The model under review builds one solid part; all positions refer to its coordinate system, in mm. Round coordinates to 2 decimals unless told otherwise and drop trailing zeros.
```python
from build123d import *

# Parameters (mm, degrees)
SKETCH3_R           = 2.201333333
SKETCH3_R_2         = 1.693333333
BOSS_EXTRUDE1_DEPTH = 914.4
CUT_EXTRUDE1_DEPTH  = 733.425


with BuildPart() as part:
    # Sketch3 → Boss-Extrude1 (new, symmetric)
    with BuildSketch(Plane.XY):
        with BuildLine():
            Line((-1.778, 0), (-1.778, 1.27))
            ThreePointArc((-1.778, 1.27), (-1.536070654, 2.494011801), (-0.846666667, 3.533942971))
            Line((-0.846666667, 3.533942971), (2.413267273, 6.793876912))
            ThreePointArc((2.413267273, 6.793876912), (2.578074335, 6.903997469), (2.772477518, 6.942666667))
            Line((2.772477518, 6.942666667), (3.048, 6.942666667))
            ThreePointArc((3.048, 6.942666667), (3.467078619, 6.769078619), (3.640666667, 6.35))
            Line((3.640666667, 6.35), (3.640666667, 4.301066667))
            ThreePointArc((3.640666667, 4.301066667), (3.948165494, 3.558698827), (4.690533333, 3.2512))
            Line((4.690533333, 3.2512), (5.300133333, 3.2512))
            ThreePointArc((5.300133333, 3.2512), (6.042501173, 3.558698827), (6.35, 4.301066667))
            Line((6.35, 4.301066667), (6.35, 10.583333333))
            ThreePointArc((6.35, 10.583333333), (5.730042687, 12.080042687), (4.233333333, 12.7))
            Line((4.233333333, 12.7), (-4.233333333, 12.7))
            ThreePointArc((-4.233333333, 12.7), (-5.730042687, 12.080042687), (-6.35, 10.583333333))
            Line((-6.35, 10.583333333), (-6.35, 0))
            Line((-6.35, 0), (-1.778, 0))
        make_face()
        with Locations(Location((-2.116666667, 8.466666667, 0), (0, 0, 180))):
            Circle(SKETCH3_R, mode=Mode.SUBTRACT)
        with Locations(Location((3.429, 9.906, 0), (0, 0, 180))):
            Circle(SKETCH3_R_2, mode=Mode.SUBTRACT)
    extrude(amount=BOSS_EXTRUDE1_DEPTH, both=True)

    # Mirror1: part across plane


with BuildPart() as part_1:
    add(part.part)
    add(part.part.mirror(Plane.ZX))

    # Sketch4 → Cut-Extrude1 (cut)
    with BuildSketch(Plane.XY.offset(914.4)):
        with BuildLine():
            Line((-6.35, 10.583333333), (-6.35, -10.583333333))
            ThreePointArc((-6.35, -10.583333333), (-5.730042687, -12.080042687), (-4.233333333, -12.7))
            Line((-4.233333333, -12.7), (4.233333333, -12.7))
            ThreePointArc((4.233333333, -12.7), (5.730042687, -12.080042687), (6.35, -10.583333333))
            Line((6.35, -10.583333333), (6.35, -4.301066667))
            ThreePointArc((6.35, -4.301066667), (6.042501173, -3.558698827), (5.300133333, -3.2512))
            Line((5.300133333, -3.2512), (4.690533333, -3.2512))
            ThreePointArc((4.690533333, -3.2512), (3.948165494, -3.558698827), (3.640666667, -4.301066667))
            Line((3.640666667, -4.301066667), (3.640666667, -6.35))
            ThreePointArc((3.640666667, -6.35), (3.467078619, -6.769078619), (3.048, -6.942666667))
            Line((3.048, -6.942666667), (2.772477518, -6.942666667))
            ThreePointArc((2.772477518, -6.942666667), (2.578074335, -6.903997469), (2.413267273, -6.793876912))
            Line((2.413267273, -6.793876912), (-0.846666667, -3.533942971))
            ThreePointArc((-0.846666667, -3.533942971), (-1.536070654, -2.494011801), (-1.778, -1.27))
            Line((-1.778, -1.27), (-1.778, 1.27))
            ThreePointArc((-1.778, 1.27), (-1.536070654, 2.494011801), (-0.846666667, 3.533942971))
            Line((-0.846666667, 3.533942971), (2.413267273, 6.793876912))
            ThreePointArc((2.413267273, 6.793876912), (2.578074335, 6.903997469), (2.772477518, 6.942666667))
            Line((2.772477518, 6.942666667), (3.048, 6.942666667))
            ThreePointArc((3.048, 6.942666667), (3.467078619, 6.769078619), (3.640666667, 6.35))
            Line((3.640666667, 6.35), (3.640666667, 4.301066667))
            ThreePointArc((3.640666667, 4.301066667), (3.948165494, 3.558698827), (4.690533333, 3.2512))
            Line((4.690533333, 3.2512), (5.300133333, 3.2512))
            ThreePointArc((5.300133333, 3.2512), (6.042501173, 3.558698827), (6.35, 4.301066667))
            Line((6.35, 4.301066667), (6.35, 10.583333333))
            ThreePointArc((6.35, 10.583333333), (5.730042687, 12.080042687), (4.233333333, 12.7))
            Line((4.233333333, 12.7), (-4.233333333, 12.7))
            ThreePointArc((-4.233333333, 12.7), (-5.730042687, 12.080042687), (-6.35, 10.583333333))
        make_face()
    extrude(amount=-CUT_EXTRUDE1_DEPTH, mode=Mode.SUBTRACT)


solid = part_1.part
```
(1) Insertion check: pin 1 (2.5 mm diameter, centred on x = -2.12, y = 8.47, fed in from -Z); pin 2 (0.5 mm diameter, centred on x = 5, z = -112.5, fed in from +Y); pin 3 (2 mm diameter, centred on y = 0.5, z = -154, fed in from +X); pin 4 (0.5 mm diameter, centred on x = 5, z = -575, fed in from -Y). Each pin has a flat end and moves straight along its axis. Give the tip position at first contact, or say it passes through.
Data:
pin 1: passes through
pin 2: stops at y = 12.64
pin 3: stops at x = -1.77
pin 4: stops at y = -12.64
(2) Consider section A-A (z = 90). State how many separate pieces and enclosed holes the cut face has, and give its area (3 significant figures).
Data:
separate pieces: 1
enclosed holes: 4
area: 196 mm2
(3) To check wall thickness, follow probe 1 along Y at (x, z) = (-3, -79); probe 2 along Y at (x, z) = (2.75, -748.5); probe 3 along Y at (x, z) = (-2.25, -284.5). State the ranges of each line that lie inside material, in increasing order.
Data:
probe 1: y = -12.7 to -10.48, -6.45 to 6.45, 10.48 to 12.7
probe 2: y = -12.7 to -11.46, -8.35 to -6.94, 6.94 to 8.35, 11.46 to 12.7
probe 3: y = -12.7 to -10.66, -6.27 to 6.27, 10.66 to 12.7
